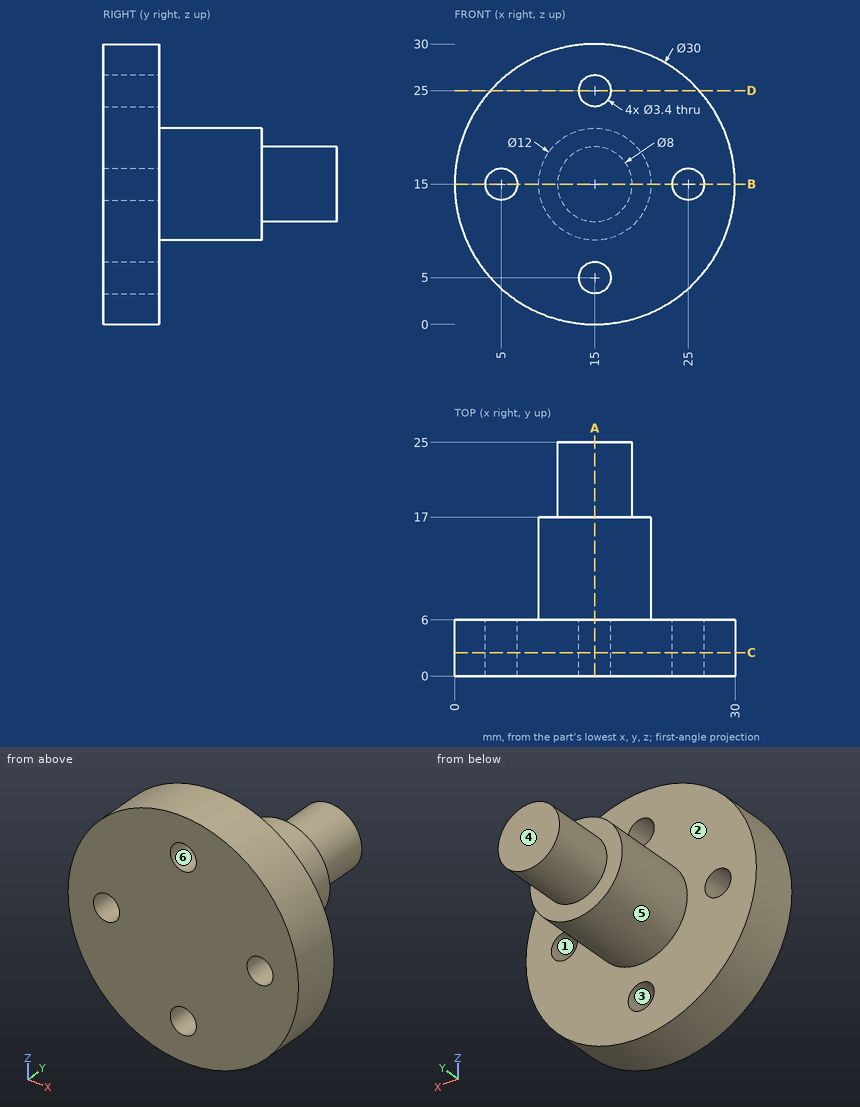
Geometry: see drawing. Coordinates: mm, zero at the bounding-box minimum. A direction names the side the tool comes from. Give positions to 0.01 mm unless a question says otherwise; leave off trailing zeros. Write each loop counter-clockwise with the first axis right and the second up, starting at its lowest first coordinate (ties: lowest second). Pieces come first, ordered by that corner, then holes. Notation, with made-up numbers: M -15.5,45 L 36.5,45 A30 ccw 36.5,76 Z; hole C 0.5,55.5 d4. An arc over 180 degrees is marked long. Return JSON: item names as keys, results as strings. Group by question number.
1) Draft query along Z for the marked faces 3, 4, 5 and 6. Return one class per face: released by +Z, released by -Z, zero draft, split by the parting line, or undercut.
2) Ray query, L1, parallel to Z at x = 15, y = 2.8; L2, parallel to Y at x = 20.25, z = 15.75; L3, parallel to Y at x = 23.25, z = 18.5. Return the intervals inside material, ascending.
3) Cut plane C-C, the plane y = 2.5. Output: boundary loops of the cut face in (x, z), then the cut area to 3 significant figures.
4) First-contact query: pin 1 Ø15 at (x, z) = (17.5, 21) entering from +Y; pin 2 Ø12 at (y, z) = (13.5, 16) entering from -X; pin 3 Ø2 at (x, z) = (26.5, 21) entering from +Y; pin 4 Ø4 at (x, y) = (8.5, 10) entering from +Z. Flat tips, straight axial feed; report the tip coordinate or a pass-through.
5) Cut plane D-D, the plane z = 25. Output: boundary loops of the cut face in (x, y), then the cut area to 3 significant figures.
6) Cut plane B-B, the plane z = 15. Output: boundary loops of the cut face in (x, y).
7) Cut plane A-A, the plane x = 15. Output: boundary loops of the cut face in (y, z), then the cut area to 3 significant figures.
8) Set-up query: the marked faces 1 and 2. Return all of +Z, -Z, +X, -X, +Y, -Y with unobstructed straight access to the full face (end or side cutting, diameter ignored); none if empty.
Data:
{
 "1": {"face 3": "undercut", "face 4": "zero draft", "face 5": "split by the parting line", "face 6": "undercut"},
 "2": {"L1": "z = 0 to 3.3, 6.7 to 23.3, 26.7 to 30", "L2": "y = 0 to 17", "L3": "y = 0 to 6"},
 "3": {"outline": "C 15,15 d30; hole C 5,15 d3.4; hole C 15,5 d3.4; hole C 15,25 d3.4; hole C 25,15 d3.4", "area": "671 mm²"},
 "4": {"pin 1": "stops at y = 25", "pin 2": "stops at x = 9", "pin 3": "stops at y = 6", "pin 4": "stops at z = 18.97"},
 "5": {"outline": "M 3.82,0 L 13.3,0 L 13.3,6 L 3.82,6 Z; M 16.7,0 L 26.18,0 L 26.18,6 L 16.7,6 Z", "area": "114 mm²"},
 "6": {"outline": "M 0,0 L 3.3,0 L 3.3,6 L 0,6 Z; M 6.7,0 L 23.3,0 L 23.3,6 L 21,6 L 21,17 L 19,17 L 19,25 L 11,25 L 11,17 L 9,17 L 9,6 L 6.7,6 Z; M 26.7,0 L 30,0 L 30,6 L 26.7,6 Z"},
 "7": {"outline": "M 0,0 L 6,0 L 6,3.3 L 0,3.3 Z; M 0,6.7 L 6,6.7 L 6,9 L 17,9 L 17,11 L 25,11 L 25,19 L 17,19 L 17,21 L 6,21 L 6,23.3 L 0,23.3 Z; M 0,26.7 L 6,26.7 L 6,30 L 0,30 Z", "area": "335 mm²"},
 "8": {"face 1": "+Y, -Y", "face 2": "+Y"}
}
